```python
from build123d import *

# Parameters (mm, degrees)
SKETCH_1_W      = 15
SKETCH_1_H      = 50
EXTRUDE_1_DEPTH = 10
FILLET_1_R      = 2
FILLET_2_R      = 2
EXTRUDE_3_DEPTH = 5
FILLET_3_R      = 2


with BuildPart() as part:
    # 스케치1 → 보스-돌출1 (new body)
    with BuildSketch(Plane(origin=(0, 0, 0), x_dir=(1, 0, 0), z_dir=(0, 1, 0))):
        Rectangle(SKETCH_1_W, SKETCH_1_H)
    extrude(amount=EXTRUDE_1_DEPTH)

    # 필렛1
    fillet_1_edges = [part.edges().sort_by_distance(p)[0] for p in [
        (7.5, 10, 0),
        (0, 10, -25),
        (-7.5, 10, 0),
        (0, 10, 25),
    ]]
    fillet(fillet_1_edges, radius=FILLET_1_R)

    # 필렛2
    # the kernel refuses this fillet: 2 mm, written as the material it takes off along each edge
    with BuildSketch(Plane(origin=(-5.5, 8, 23), x_dir=(-1, 0, 0), z_dir=(0, 0, 1))) as fillet_2_piece_1_section:
        Polygon((0, 0), (FILLET_2_R, 0), (FILLET_2_R, -FILLET_2_R), (0, -FILLET_2_R), align=None)
    fillet_2_piece_1 = extrude(amount=FILLET_2_R, mode=Mode.PRIVATE)
    fillet_2_piece_1 = fillet_2_piece_1 - Plane(origin=(-5.5, 8, 23), x_dir=(0.7071067811865475, -0.7071067811865475, 0), z_dir=(0, 0, 1)) * Sphere(FILLET_2_R, mode=Mode.PRIVATE)
    add(fillet_2_piece_1, mode=Mode.SUBTRACT)
    with BuildSketch(Plane(origin=(-5.5, 8, -23), x_dir=(0, 0, -1), z_dir=(-1, 0, 0))) as fillet_2_piece_2_section:
        Polygon((0, 0), (FILLET_2_R, 0), (FILLET_2_R, -FILLET_2_R), (0, -FILLET_2_R), align=None)
    fillet_2_piece_2 = extrude(amount=FILLET_2_R, mode=Mode.PRIVATE)
    fillet_2_piece_2 = fillet_2_piece_2 - Plane(origin=(-5.5, 8, -23), x_dir=(0, -0.7071067811865475, 0.7071067811865475), z_dir=(-1, 0, 0)) * Sphere(FILLET_2_R, mode=Mode.PRIVATE)
    add(fillet_2_piece_2, mode=Mode.SUBTRACT)
    with BuildSketch(Plane(origin=(5.5, 8, 23), x_dir=(1, 0, 0), z_dir=(0, 0, 1))) as fillet_2_piece_3_section:
        Polygon((0, 0), (FILLET_2_R, 0), (FILLET_2_R, FILLET_2_R), (0, FILLET_2_R), align=None)
    fillet_2_piece_3 = extrude(amount=FILLET_2_R, mode=Mode.PRIVATE)
    fillet_2_piece_3 = fillet_2_piece_3 - Plane(origin=(5.5, 8, 23), x_dir=(-0.7071067811865475, -0.7071067811865475, 0), z_dir=(0, 0, 1)) * Sphere(FILLET_2_R, mode=Mode.PRIVATE)
    add(fillet_2_piece_3, mode=Mode.SUBTRACT)
    with BuildSketch(Plane(origin=(5.5, 8, -23), x_dir=(0, 0, -1), z_dir=(1, 0, 0))) as fillet_2_piece_4_section:
        Polygon((0, 0), (FILLET_2_R, 0), (FILLET_2_R, FILLET_2_R), (0, FILLET_2_R), align=None)
    fillet_2_piece_4 = extrude(amount=FILLET_2_R, mode=Mode.PRIVATE)
    fillet_2_piece_4 = fillet_2_piece_4 - Plane(origin=(5.5, 8, -23), x_dir=(0, -0.7071067811865475, 0.7071067811865475), z_dir=(1, 0, 0)) * Sphere(FILLET_2_R, mode=Mode.PRIVATE)
    add(fillet_2_piece_4, mode=Mode.SUBTRACT)
    with BuildSketch(Plane(origin=(7.5, -5, -25), x_dir=(0, 0, 1), z_dir=(0, 1, 0)), Plane(origin=(7.5, -5, 25), x_dir=(-1, 0, 0), z_dir=(0, 1, 0))) as fillet_2_piece_5:
        with BuildLine():
            CenterArc((FILLET_2_R, -FILLET_2_R), FILLET_2_R, 90, 90)
            Line((0, -FILLET_2_R), (0, 0))
            Line((0, 0), (FILLET_2_R, 0))
        make_face()
    extrude(amount=13, mode=Mode.SUBTRACT)
    with BuildSketch(Plane(origin=(-7.5, -5, 25), x_dir=(1, 0, 0), z_dir=(0, 1, 0)), Plane(origin=(-7.5, -5, -25), x_dir=(0, 0, 1), z_dir=(0, 1, 0))) as fillet_2_piece_6:
        with BuildLine():
            CenterArc((FILLET_2_R, FILLET_2_R), FILLET_2_R, 180, 90)
            Line((0, FILLET_2_R), (0, 0))
            Line((0, 0), (FILLET_2_R, 0))
        make_face()
    extrude(amount=13, mode=Mode.SUBTRACT)

    # 스케치4 → 보스-돌출3 (add, symmetric)
    with BuildSketch(Plane(origin=(0, 0, 0), x_dir=(0, 0, -1), z_dir=(1, 0, 0))):
        with BuildLine():
            Line((20, 0), (-20, 0))
            Line((-20, 0), (-20, 104))
            Line((-20, 104), (-20, 124))
            ThreePointArc((-20, 124), (0, 104), (20, 124))
            Line((20, 124), (20, 104))
            Line((20, 104), (20, 0))
        make_face()
    extrude(amount=EXTRUDE_3_DEPTH, both=True)

    # 필렛3
    fillet_3_edges = [part.edges().sort_by_distance(p)[0] for p in [
        (0, 10, -20),
        (0, 10, 20),
    ]]
    fillet(fillet_3_edges, radius=FILLET_3_R)


solid = part.part
```
Read the model definition and answer for the solid it produces. Units are mm, in the model's axes. A direction names the side the tool comes from. Give positions to 0.01 mm unless a question says otherwise; leave off trailing zeros. Write each loop counter-clockwise with the first axis right and the second up, starting at its lowest first coordinate (ties: lowest second). Pieces come first, ordered by that corner, then holes. Notation, with made-up numbers: M 4.5,83 L 49.5,83 A9 cw 49.5,91 Z; hole C 54.5,-37 d1. An arc over 180 degrees is marked long. Put each result on its own line as item: value. Start each with the question number.
1. The part is cut by section B-B, the plane x = 2.25. Give the vertices of the cut face in (y, z).
2. For a pull along Z with two mould halves and no side action, classify faces 6 (the flat face through (0, 4, 25)), 7 (the flat face through (-5, 55, 0)), 8 (the cylindrical face through (0, 104, 0)), 9 (the flat face through (0, 4, -25)) as released by +Z, released by -Z, zero draft, split by the parting line, or undercut.
3. The part is cut by section C-C, the plane y = 73. Give the vertices of the cut face in (x, z), and give its area (3 significant figures).
4. Which of the six approach directions +Z, -Z, +X, -X, +Y, -Y give full straight-line access (tool end or side, diameter ignored) to faces 1 (the flat face through (5, 55, 0)), 2 (the flat face through (0, 67, 20)), 3 (the flat face through (7.5, 4, 0)), 4 (the flat face through (-5.3, 10, -0.1)), 5 (the flat face through (0, 69, -20))?
5. Consider line 1 along X through (y, z) = (16.5, 11.5); line 2 along Z through (x, y) = (-4, 36); line 3 along Y through (x, z) = (-3, -23). Determine where each line is inside the solid, lowest interval first.
6. The part is cut by section D-D, the plane z = -11.5. Give the vertices of the cut face in (x, y), and give its area (3 significant figures).
7. Each of these flat-tipped pins is pushed along its axis until it touches: pin 1 Ø1 at (y, z) = (97, 13) entering from +X; pin 2 Ø4 at (y, z) = (85.5, -17) entering from -X; pin 3 Ø3 at (x, y) = (-2, 69.5) entering from -Z. Where does it stop, or does it pass through?
8. The part is cut by section A-A, the plane z = 0. Give the vertices of the cut face in (x, y), and give its area (3 significant figures).
Final values:
1. outline: M 0,-25 L 8,-25 A2 ccw 10,-23 L 10,-22 A2 cw 12,-20 L 124,-20 A20 cw 124,20 L 12,20 A2 cw 10,22 L 10,23 A2 ccw 8,25 L 0,25 Z
2. face 6: released by +Z
2. face 7: zero draft
2. face 8: undercut
2. face 9: released by -Z
3. outline: M -5,-20 L 5,-20 L 5,20 L -5,20 Z
3. area: 400 mm²
4. face 1: +Z, -Z, +X, +Y
4. face 2: +Z, +X, -X, +Y
4. face 3: +Z, -Z, +X, +Y, -Y
4. face 4: +Y
4. face 5: -Z, +X, -X, +Y
5. line 1: x = -5 to 5
5. line 2: z = -20 to 20
5. line 3: y = 0 to 10
6. outline: M -7.5,0 L 7.5,0 L 7.5,8 A2 ccw 5.5,10 L 5,10 L 5,107.64 L -5,107.64 L -5,10 L -5.5,10 A2 ccw -7.5,8 Z
6. area: 1,120 mm²
7. pin 1: stops at x = 5
7. pin 2: stops at x = -5
7. pin 3: stops at z = -20
8. outline: M -7.5,0 L 7.5,0 L 7.5,8 A2 ccw 5.5,10 L 5,10 L 5,104 L -5,104 L -5,10 L -5.5,10 A2 ccw -7.5,8 Z
8. area: 1,090 mm²
